Design review of the part built by this model. Coordinates are the model's own, in mm. A direction names the side the tool comes from. Give positions to 0.01 mm unless a question says otherwise; leave off trailing zeros. Order: outer loops, then holes, each group sorted by start corner. A loop starts at its lowest first (then second) coordinate and runs counter-clockwise, first axis right, second up. Notation, with made-up numbers: (-26, 67) -> (12, 67) arc R20 cw to (12, 93) -> close; hole circle Ø10 at (70.25, -21.75). An arc over 180 degrees is marked (long way). One line per item, written item: value.
from build123d import *

# Parameters (mm, degrees)
SKETCH_1_R          = 16
SKETCH_1_R_2        = 2.25
EXTRUDE_1_DEPTH     = 8
CUT_EXTRUDE_1_DEPTH = 6.8
CUT_EXTRUDE_8_DEPTH = 1


with BuildPart() as part:
    # Эскиз1 → Бобышка-Вытянуть1 (new body)
    with BuildSketch(Plane(origin=(0, 0, 0), x_dir=(1, 0, 0), z_dir=(0, 1, 0))):
        with BuildLine():
            Line((-27.5, -25.4), (-7.5, -25.4))
            Line((-7.5, -25.4), (-7.5, -22.955849111))
            ThreePointArc((-7.5, -22.955849111), (-6.68281162, -21.343100938), (-4.899043329, -21.048271831))
            ThreePointArc((-4.899043329, -21.048271831), (4.948796089, -21.832347138), (14.151976117, -18.241220202))
            ThreePointArc((14.151976117, -18.241220202), (14.777726241, -18.069792078), (15.376980036, -18.318480053))
            Line((15.376980036, -18.318480053), (17.814747272, -20.472785982))
            ThreePointArc((17.814747272, -20.472785982), (22.472785982, -20.185252728), (22.185252728, -15.527214018))
            Line((22.185252728, -15.527214018), (20.143734708, -13.723081814))
            ThreePointArc((20.143734708, -13.723081814), (19.813719174, -13.098302749), (19.979075206, -12.411340949))
            ThreePointArc((19.979075206, -12.411340949), (22.823148445, -6.493089604), (23.8, 0))
            ThreePointArc((23.8, 0), (9.576401492, 22.98111988), (-17.333078903, 20.466663618))
            ThreePointArc((-17.333078903, 20.466663618), (-17.974550182, 20.264645495), (-18.598905377, 20.514600122))
            Line((-18.598905377, 20.514600122), (-20.814747272, 22.472785982))
            ThreePointArc((-20.814747272, 22.472785982), (-25.472785982, 22.185252728), (-25.185252728, 17.527214018))
            Line((-25.185252728, 17.527214018), (-23.20688118, 15.778885673))
            ThreePointArc((-23.20688118, 15.778885673), (-22.876796583, 15.153555184), (-23.04284729, 14.466226133))
            ThreePointArc((-23.04284729, 14.466226133), (-26.362874376, 7.569397218), (-27.5, 0))
            Line((-27.5, 0), (-27.5, -25.4))
        make_face()
        Circle(SKETCH_1_R, mode=Mode.SUBTRACT)
        with Locations((-23, 20)):
            Circle(SKETCH_1_R_2, mode=Mode.SUBTRACT)
        with Locations((20, -18)):
            Circle(SKETCH_1_R_2, mode=Mode.SUBTRACT)
    extrude(amount=-EXTRUDE_1_DEPTH)

    # Эскиз2 → Вырез-Вытянуть1 (cut)
    with BuildSketch(Plane(origin=(0, -8, 0), x_dir=(-1, 0, 0), z_dir=(0, -1, 0))):
        with BuildLine():
            Line((8.5, -25.4), (8.5, -22.955849111))
            ThreePointArc((8.5, -22.955849111), (7.274217431, -20.536726851), (4.598564994, -20.094483191))
            ThreePointArc((4.598564994, -20.094483191), (-4.803026036, -20.843028639), (-13.589169994, -17.414631267))
            ThreePointArc((-13.589169994, -17.414631267), (-16.632858543, -14.893819788), (-19.152217909, -11.84892917))
            ThreePointArc((-19.152217909, -11.84892917), (-21.867461922, -6.198703298), (-22.799999997, 0.000326884))
            ThreePointArc((-22.799999997, 0.000326884), (-9.131074658, 22.085751778), (16.729450225, 19.669398029))
            ThreePointArc((16.729450225, 19.669398029), (19.707335368, 17.009099388), (22.216615604, 13.902895678))
            ThreePointArc((22.216615604, 13.902895678), (25.407255273, 7.274792502), (26.500000107, 0.000327424))
            Line((26.500000107, 0.000327424), (26.5, -25.4))
            Line((26.5, -25.4), (8.5, -25.4))
        make_face()
    extrude(amount=-CUT_EXTRUDE_1_DEPTH, mode=Mode.SUBTRACT)

    # Эскиз11 → Вырез-Вытянуть8 (cut)
    with BuildSketch(Plane.XZ.offset(8)):
        with BuildLine():
            Line((-8.5, 22.955849111), (-8.5, 25.4))
            Line((-8.5, 25.4), (-8, 25.4))
            Line((-8, 25.4), (-8, 22.955849111))
            ThreePointArc((-8, 22.955849111), (-6.978514526, 20.939913894), (-4.748804162, 20.571377511))
            ThreePointArc((-4.748804162, 20.571377511), (14.487462515, 17.39189423), (23.3, -0.000122694))
            ThreePointArc((23.3, -0.000122694), (-1.849981151, -25.16680236), (-26.999999983, -0.000160392))
            Line((-26.999999983, -0.000160392), (-27.000000053, 25.4))
            Line((-27.000000053, 25.4), (-26.500000054, 25.4))
            Line((-26.500000054, 25.4), (-26.500000053, -0.000327424))
            ThreePointArc((-26.500000053, -0.000327424), (-1.849999809, -24.666802429), (22.799999998, -0.000327043))
            ThreePointArc((22.799999998, -0.000327043), (14.191842001, 16.98864676), (-4.598564994, 20.094483191))
            ThreePointArc((-4.598564994, 20.094483191), (-7.274217431, 20.536726851), (-8.5, 22.955849111))
        make_face()
    extrude(amount=-CUT_EXTRUDE_8_DEPTH, mode=Mode.SUBTRACT)


solid = part.part
Item 1: To check wall thickness, follow line 1 along X through (y, z) = (-7.5, 17); line 2 along Z through (x, y) = (20, -6); line 3 along Z through (x, y) = (-23, -1). State the ranges of each line that lie inside material, in increasing order. Write a range as from..to.
Returned:
line 1: -27.5..-27, 15.01..17.98, 22.02..23.14
line 2: -13.45..-11.43, 10.49..12.38, 13.57..15.75, 20.25..21.3
line 3: -23.3..-22.25, -17.75..-15.52, -14.53..25.4
Item 2: Add section D-D on x = 8. Give the boundary of the cut face in (y, z).
Returned:
outline: (-8, -23.7) -> (0, -23.7) -> (0, -13.86) -> (-1.2, -13.86) -> (-1.2, -22.61) -> (-7, -22.61) -> (-7, -23.16) -> (-8, -23.16) -> close; (-8, 20.64) -> (-7, 20.64) -> (-7, 20.11) -> (-1.2, 20.11) -> (-1.2, 13.86) -> (0, 13.86) -> (0, 21.16) -> (-8, 21.16) -> close
Item 3: Machinability: for faces 5 (the flat face through (-24.21, -3.944, -16.665)), 6 (the flat face through (-26.5, -4, 13)), 7 (the flat face through (16.6, -3.9, 19.4)), which of the approach directions +Z, -Z, +X, -X, +Y, -Y give a long, thin tool a straight path to every point of the face, cutting with its end or side? Answer none if there is none.
Returned:
face 5: -X, +Y, -Y
face 6: +Z, -Y
face 7: +Z, +Y, -Y
Item 4: Clearance check with flat-ended pins moving along their axes: P1, Ø2.5, axis at y = -4.5, z = 24.5, coming from the +X side; P2, Ø2, axis at y = -7, z = 6, coming from the +X side; P3, Ø5, axis at x = 20, z = 18, coming from the -Y side; P4, Ø2, axis at x = -17.5, y = -6.5, coming from the -Z side. State where each tip first meets the part, or that it passes through.
Returned:
P1: x = -7.5
P2: x = 23.23
P3: y = -8
P4: z = -21.07
Item 5: Add section B-B on x = -11. Give the boundary of the cut face in (y, z), plus the area to 3 significant figures.
Returned:
outline: (-8, -23.98) -> (0, -23.98) -> (0, -11.62) -> (-1.2, -11.62) -> (-1.2, -22.91) -> (-7, -22.91) -> (-7, -23.44) -> (-8, -23.44) -> close; (-1.2, 11.62) -> (0, 11.62) -> (0, 25.4) -> (-1.2, 25.4) -> close
area: 38.1 mm²
Item 6: Add section A-A on z = 9. Give the boundary of the cut face in (x, y).
Returned:
outline: (-27.5, -8) -> (-27, -8) -> (-27, -7) -> (-26.5, -7) -> (-26.5, -1.2) -> (-13.23, -1.2) -> (-13.23, 0) -> (-27.5, 0) -> close; (13.23, -1.2) -> (20.78, -1.2) -> (20.78, -7) -> (21.33, -7) -> (21.33, -8) -> (21.88, -8) -> (21.88, 0) -> (13.23, 0) -> close
Item 7: Draft analysis for pull direction X (two halves, no side actions). For faces 1 (the flat face through (23, -8, 5)), 2 (the cylindrical face through (-7.306, -4.141, 20.56)), 3 (the flat face through (-27.5, -4, 13)), 4 (the cylindrical face through (22.796, -3.944, 6.581)), state which applies: pulls with the +X half, pulls with the -X half, needs draft (parallel to the pull), parting line crosses it, or undercut.
Returned:
face 1: needs draft
face 2: undercut
face 3: pulls with the -X half
face 4: pulls with the +X half
Item 8: Add section C-C on y = -3.5. Give the boundary of the cut face in (x, z), plus the area to 3 significant figures.
Returned:
outline: (-27.5, 0) arc R25.65 ccw to (-23.04, -14.47) arc R1 cw to (-23.21, -15.78) -> (-25.19, -17.53) arc R3.3 ccw to (-20.81, -22.47) -> (-18.6, -20.51) arc R1 cw to (-17.33, -20.47) arc R25.65 ccw to (23.8, 0) arc R22.07 ccw to (19.98, 12.41) arc R1 cw to (20.14, 13.72) -> (22.19, 15.53) arc R3.3 ccw to (17.81, 20.47) -> (15.38, 18.32) arc R1 cw to (14.15, 18.24) arc R22.07 ccw to (-4.9, 21.05) arc R2 cw to (-7.5, 22.96) -> (-7.5, 25.4) -> (-8.5, 25.4) -> (-8.5, 22.96) arc R3 ccw to (-4.6, 20.09) arc R21.07 cw to (22.8, 0) arc R24.65 cw to (-22.22, -13.9) arc R24.65 cw to (-26.5, 0) -> (-26.5, 25.4) -> (-27.5, 25.4) -> close; hole circle Ø4.5 at (-23, -20); hole circle Ø4.5 at (20, 18)
area: 202 mm²
